Can you work these out from the model? Positions are in its coordinate system, mm. A direction names the side the tool comes from. Give positions to 0.01 mm unless a question says otherwise; leave off trailing zeros. Write each loop counter-clockwise with the first axis right and the second up, starting at its lowest first coordinate (ties: lowest second). Pieces come first, ordered by that corner, then holes.
1. Thinking about a two-plate mould opening in Y: for faces 1 (the flat face through (12, 30.099, -1)), 2 (the cylindrical face through (1.94, 3.93, -0.79)), 3 (the flat face through (11, 12, 8.38)), which applies, pulls with the +Y half, pulls with the -Y half, needs draft (parallel to the pull), parting line crosses it, or undercut?
2. Suppose I cut it at C-C (y = 9). Please give me the cut outline in (x, z), and give its area (3 significant figures).
3. Suppose I cut it at B-B (x = 3.5). Please give me the cut outline in (y, z).
4. On a 3-axis mill with a long thin cutter (end or side, diameter ignored), from which of +Z, -Z, +X, -X, +Y, -Y can I reach the whole of each face in a straight line? I mean faces 4 (the flat face through (12, 15, -1.6)), 5 (the flat face through (14, 12, 8.38)), 6 (the flat face through (12, 10.71, 1)), 7 (the cylindrical face through (14.05, 11.08, 5.42)), 8 (the cylindrical face through (14.05, 11.08, -0.79)). Say none if no direction works.
5. If I drill on probe 1 along Z at (x, y) = (8.5, 14); probe 2 along Y at (x, z) = (10, 1.25); probe 3 along X at (y, z) = (26.5, -0.5), over which ranges is the centre line in solid material (lowest first)?
6. Suppose I cut it at D-D (z = 3.5). Please give me the cut outline in (x, y) (3 decimals).
7. Suppose I cut it at A-A (x = 17.75). Please give me the cut outline in (y, z), and give its area (3 significant figures).
8. I'm going to push flat-ended pins straight in: pin 1 (1.8 mm diameter, centred on x = 21.336, y = 2.921, fed in from -Z); pin 2 (1.6 mm diameter, centred on x = 13.65, y = 14.39, fed in from -Z); pin 3 (5 mm diameter, centred on x = 15.5, y = 24, fed in from +Z); pin 4 (2 mm diameter, centred on y = 13.5, z = 1.5, fed in from -X). Where does each tip first touch, or does it pass through?
```python
from build123d import *

# Parameters (mm, degrees)
SKETCH1_W           = 24.13
SKETCH1_H           = 30.099
SKETCH1_R           = 1.5
SKETCH1_R_2         = 0.875
BOSS_EXTRUDE1_DEPTH = 1.6
SKETCH1_19_W        = 5.08
SKETCH1_19_H        = 4.83
SKETCH1_19_R        = 0.875
BOSS_EXTRUDE2_DEPTH = 2.54
SKETCH1_20_R        = 0.875
BOSS_EXTRUDE3_DEPTH = 8.38


with BuildPart() as part:
    # Sketch1 → Boss-Extrude1 (new body)
    with BuildSketch(Plane.XY):
        with Locations((12.065, 15.0495)):
            Rectangle(SKETCH1_W, SKETCH1_H)
        with Locations((3.048, 2.921)):
            Circle(SKETCH1_R, mode=Mode.SUBTRACT)
        with Locations((21.336, 2.921)):
            Circle(SKETCH1_R, mode=Mode.SUBTRACT)
        with Locations((3.048, 27.051)):
            Circle(SKETCH1_R, mode=Mode.SUBTRACT)
        with Locations((6.908038, 13.09497)):
            Circle(SKETCH1_R, mode=Mode.SUBTRACT)
        with Locations((18.008092, 13.09497)):
            Circle(SKETCH1_R, mode=Mode.SUBTRACT)
        with Locations((11.107928, 14.394942)):
            Circle(SKETCH1_R_2, mode=Mode.SUBTRACT)
        with Locations((13.647928, 14.394942)):
            Circle(SKETCH1_R_2, mode=Mode.SUBTRACT)
        with Locations((11.107928, 11.854942)):
            Circle(SKETCH1_R_2, mode=Mode.SUBTRACT)
        with Locations((13.647928, 11.854942)):
            Circle(SKETCH1_R_2, mode=Mode.SUBTRACT)
    extrude(amount=-BOSS_EXTRUDE1_DEPTH)

    # Sketch1_19 → Boss-Extrude2 (add)
    with BuildSketch(Plane.XY):
        with Locations((12.377928, 13.124942)):
            Rectangle(SKETCH1_19_W, SKETCH1_19_H)
        with Locations((13.647928, 11.854942)):
            Circle(SKETCH1_19_R, mode=Mode.SUBTRACT)
        with Locations((11.107928, 11.854942)):
            Circle(SKETCH1_19_R, mode=Mode.SUBTRACT)
        with Locations((13.647928, 14.394942)):
            Circle(SKETCH1_19_R, mode=Mode.SUBTRACT)
        with Locations((11.107928, 14.394942)):
            Circle(SKETCH1_19_R, mode=Mode.SUBTRACT)
        with Locations((13.647928, 11.854942)):
            Circle(SKETCH1_19_R)
        with Locations((11.107928, 11.854942)):
            Circle(SKETCH1_19_R)
        with Locations((11.107928, 14.394942)):
            Circle(SKETCH1_19_R)
        with Locations((13.647928, 14.394942)):
            Circle(SKETCH1_19_R)
    extrude(amount=BOSS_EXTRUDE2_DEPTH)

    # Sketch1_20 → Boss-Extrude3 (add)
    with BuildSketch(Plane.XY):
        with Locations((13.647928, 14.394942)):
            Circle(SKETCH1_20_R)
        with Locations((11.107928, 14.394942)):
            Circle(SKETCH1_20_R)
        with Locations((11.107928, 11.854942)):
            Circle(SKETCH1_20_R)
        with Locations((13.647928, 11.854942)):
            Circle(SKETCH1_20_R)
    extrude(amount=BOSS_EXTRUDE3_DEPTH)


solid = part.part
```
Checks:
1. face 1: pulls with the +Y half
1. face 2: undercut
1. face 3: needs draft
2. outline: (0, -1.6) - (24.13, -1.6) - (24.13, 0) - (0, 0) - close
2. area: 38.6 mm2
3. outline: (0, -1.6) - (1.49, -1.6) - (1.49, 0) - (0, 0) - close; (4.35, -1.6) - (25.62, -1.6) - (25.62, 0) - (4.35, 0) - close; (28.48, -1.6) - (30.1, -1.6) - (30.1, 0) - (28.48, 0) - close
4. face 4: -Z, +X, -X, +Y, -Y
4. face 5: +Z, +X, -X, +Y, -Y
4. face 6: +Z, +X, -X, -Y
4. face 7: +Z
4. face 8: -Z
5. probe 1: z = -1.6 to 0
5. probe 2: y = 10.71 to 15.54
5. probe 3: x = 0 to 1.65, 4.44 to 24.13
6. outline: circle Ø1.75 at (11.108, 11.855); circle Ø1.75 at (11.108, 14.395); circle Ø1.75 at (13.648, 11.855); circle Ø1.75 at (13.648, 14.395)
7. outline: (0, -1.6) - (11.62, -1.6) - (11.62, 0) - (0, 0) - close; (14.57, -1.6) - (30.1, -1.6) - (30.1, 0) - (14.57, 0) - close
7. area: 43.4 mm2
8. pin 1: passes through
8. pin 2: stops at z = 0
8. pin 3: stops at z = 0
8. pin 4: stops at x = 9.84
